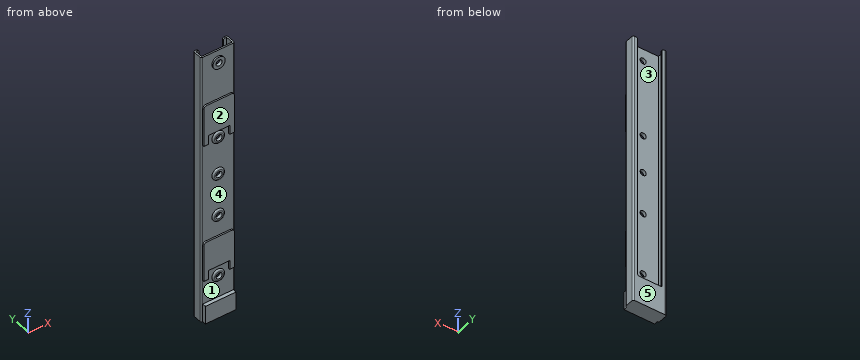
```python
from build123d import *

# Parameters (mm, degrees)
SKETCH1_W           = 11
SKETCH1_H           = 90
BOSS_EXTRUDE1_DEPTH = 3.5
CUT_EXTRUDE1_DEPTH  = 81
CUT_EXTRUDE2_DEPTH  = 6
FILLET1_R           = 0.5
FILLET2_R           = 0.5
SKETCH4_R           = 2
SKETCH4_R_2         = 1
BOSS_EXTRUDE2_DEPTH = 0.5
CUT_EXTRUDE3_START  = -1
SKETCH4_2_R         = 1
CUT_EXTRUDE3_DEPTH  = 1
FILLET3_R           = 0.5
FILLET4_R           = 1
SKETCH5_W           = 10
SKETCH5_H           = 6
BOSS_EXTRUDE3_DEPTH = 1.2


with BuildPart() as part:
    # Sketch1 → Boss-Extrude1 (new body)
    with BuildSketch(Plane(origin=(0, 0, 0), x_dir=(1, 0, 0), z_dir=(0, 1, 0))):
        Rectangle(SKETCH1_W, SKETCH1_H)
    extrude(amount=BOSS_EXTRUDE1_DEPTH)

    # Sketch2 → Cut-Extrude1 (cut)
    with BuildSketch(Plane.XY.offset(45)):
        Polygon((-4, 3.5), (-4, 3), (-5, 3), (-5, 0.5), (5, 0.5), (5, 3), (4, 3), (4, 3.5), align=None)
    extrude(amount=-CUT_EXTRUDE1_DEPTH, mode=Mode.SUBTRACT)

    # Sketch3 → Cut-Extrude2 (cut)
    with BuildSketch(Plane.XY.offset(-36)):
        Polygon((-4, 3), (4, 3), (5, 3), (5, 0.5), (-5, 0.5), (-5, 3), align=None)
    extrude(amount=-CUT_EXTRUDE2_DEPTH, mode=Mode.SUBTRACT)

    # Fillet1
    fillet1_edges = [part.edges().sort_by_distance(p)[0] for p in [
        (-5.5, 3.5, 0),
        (5.5, 3.5, 0),
        (-5.5, 0, 0),
        (5.5, 0, 0),
    ]]
    fillet(fillet1_edges, radius=FILLET1_R)

    # Fillet2
    fillet2_edges = [part.edges().sort_by_distance(p)[0] for p in [
        (4, 3.25, -36),
        (-4, 3.25, -36),
        (-4, 3.25, 45),
        (4, 3.25, 45),
    ]]
    fillet(fillet2_edges, radius=FILLET2_R)

    # Sketch4 → Boss-Extrude2 (add)
    # profile 1 of 7: a face of its own
    with BuildSketch(Plane.XZ):
        with Locations(Location((0, -31.5, 0), (0, 0, 270))):
            Circle(SKETCH4_R)
        with Locations(Location((0, -31.5, 0), (0, 0, 270))):
            Circle(SKETCH4_R_2, mode=Mode.SUBTRACT)
    # profile 2 of 7: a face of its own
    with BuildSketch(Plane.XZ):
        with Locations(Location((0, -11, 0), (0, 0, 270))):
            Circle(SKETCH4_R)
        with Locations(Location((0, -11, 0), (0, 0, 270))):
            Circle(SKETCH4_R_2, mode=Mode.SUBTRACT)
    # profile 3 of 7: a face of its own
    with BuildSketch(Plane.XZ):
        with Locations(Location((0, 3, 0), (0, 0, 270))):
            Circle(SKETCH4_R)
        with Locations(Location((0, 3, 0), (0, 0, 270))):
            Circle(SKETCH4_R_2, mode=Mode.SUBTRACT)
    # profile 4 of 7: a face of its own
    with BuildSketch(Plane.XZ):
        with Locations(Location((0, 41, 0), (0, 0, 270))):
            Circle(SKETCH4_R)
        with Locations(Location((0, 41, 0), (0, 0, 270))):
            Circle(SKETCH4_R_2, mode=Mode.SUBTRACT)
    # profile 5 of 7: a face of its own
    with BuildSketch(Plane.XZ):
        with Locations(Location((0, 15.5, 0), (0, 0, 270))):
            Circle(SKETCH4_R)
        with Locations(Location((0, 15.5, 0), (0, 0, 270))):
            Circle(SKETCH4_R_2, mode=Mode.SUBTRACT)
    # profile 6 of 7: a face of its own
    with BuildSketch(Plane.XZ):
        Polygon((5, 28.5), (-5, 28.5), (-5, 15), (-3.5, 15), (-3.5, 18), (3.5, 18), (3.5, 15), (5, 15), align=None)
    # profile 7 of 7: a face of its own
    with BuildSketch(Plane.XZ):
        Polygon((5, -18), (-5, -18), (-5, -31), (-3.5, -31), (-3.5, -28), (3.5, -28), (3.5, -31), (5, -31), align=None)
    extrude(amount=BOSS_EXTRUDE2_DEPTH)

    # Sketch4<2> → Cut-Extrude3 (cut)
    with BuildSketch(Plane.XZ.offset(CUT_EXTRUDE3_START)):
        with Locations(Location((0, -31.5, 0), (0, 0, 270))):
            Circle(SKETCH4_2_R)
        with Locations(Location((0, -11, 0), (0, 0, 270))):
            Circle(SKETCH4_2_R)
        with Locations(Location((0, 3, 0), (0, 0, 270))):
            Circle(SKETCH4_2_R)
        with Locations(Location((0, 15.5, 0), (0, 0, 270))):
            Circle(SKETCH4_2_R)
        with Locations(Location((0, 41, 0), (0, 0, 270))):
            Circle(SKETCH4_2_R)
    extrude(amount=CUT_EXTRUDE3_DEPTH, mode=Mode.SUBTRACT)

    # Fillet3
    fillet3_edges = [part.edges().sort_by_distance(p)[0] for p in [
        (0, -0.5, -29.5),
        (0, -0.5, -9),
        (0, -0.5, 5),
        (0, -0.5, 17.5),
    ]]
    fillet(fillet3_edges, radius=FILLET3_R - 0.0001)  # a hair under: the kernel refuses the full size

    # Fillet4
    fillet4_edges = [part.edges().sort_by_distance(p)[0] for p in [
        (5, -0.25, 28.5),
        (-5, -0.25, 28.5),
        (5, -0.25, -18),
        (-5, -0.25, -18),
    ]]
    fillet(fillet4_edges, radius=FILLET4_R)

    # Sketch5 → Boss-Extrude3 (add)
    with BuildSketch(Plane.XZ):
        with Locations((0, -42)):
            Rectangle(SKETCH5_W, SKETCH5_H)
    extrude(amount=BOSS_EXTRUDE3_DEPTH)


solid = part.part
```
Verification items for the finished model (mm, model axes). Face numbers are marked on the shaded views. A direction names the side the tool comes from. Coordinates: 2 decimals unless noted, no trailing zeros. Order: outer loops, then holes, each group sorted by start corner. A loop starts at its lowest first (then second) coordinate and runs counter-clockwise, first axis right, second up. Notation, with made-up numbers: (-32, -15) -> (-21, -15) arc R32 cw to (-21, 16) -> close; hole circle Ø6 at (15.25, 40.25). An arc over 180 degrees is marked (long way). Answer as CSV lines item,"result". Start each with the question number.
1) Set-up check for the marked faces 1 and 2: record each of +Z, -Z, +X, -X, +Y, -Y from which the full face is reachable in a straight line by a thin tool's end or side.
2) Cross-section at B-B, the plane y = 1.25. Record the boundary of the cut face in (x, z).
3) Release check for a two-part mould opening along Y. For the marked faces 3, 4 and 5 record: released by +Y, released by -Y, zero draft, split by the parting line, or undercut.
4) Cross-section at D-D, the plane x = 0. Give the number of separate pieces and of enclosed holes in the cut face, then the cut area to 3 significant figures.
5) Material ranges on L1, parallel to Z at x = 0, y = 0.05; L2, parallel to X at y = 1.25, z = -39; L3, parallel to X at y = -0.1, z = 3, recorded low to high. Write a range as [from, to].
6) Cross-section at A-A, the plane z = 41. Record the boundary of the cut face in (x, y).
7) Gauge pin test, flat ends, axial feed: pin 1 Ø4.5 at (x, z) = (0.5, 41.5) entering from -Y; pin 2 Ø1.3 at (y, z) = (-0.5, -41) entering from -X; pin 3 Ø3 at (x, z) = (0, -11) entering from +Y. Record the tip position at first contact, or that the pin passes through.
Conclusion:
1,face 1,"-Y"
1,face 2,"+Z, +X, -X, -Y"
2,outline,"(-5.5, -45) -> (5.5, -45) -> (5.5, 45) -> (5, 45) -> (5, -42) -> (-5, -42) -> (-5, 45) -> (-5.5, 45) -> close"
3,face 3,"undercut"
3,face 4,"released by -Y"
3,face 5,"released by +Y"
4,separate pieces,"6"
4,enclosed holes,"0"
4,area,"74.0 mm²"
5,L1,"z = [-45, -32.5], [-30.5, -12], [-10, 2], [4, 14.5], [16.5, 40], [42, 45]"
5,L2,"x = [-5.5, -5], [5, 5.5]"
5,L3,"x = [-1.99, -1], [1, 1.99]"
6,outline,"(-5.5, 0.5) arc R0.5 ccw to (-5, 0) -> (-2, 0) -> (-2, -0.5) -> (-1, -0.5) -> (-1, 0.5) -> (-5, 0.5) -> (-5, 3) -> (-4, 3) -> (-4, 3.5) -> (-5, 3.5) arc R0.5 ccw to (-5.5, 3) -> close; (1, -0.5) -> (2, -0.5) -> (2, 0) -> (5, 0) arc R0.5 ccw to (5.5, 0.5) -> (5.5, 3) arc R0.5 ccw to (5, 3.5) -> (4, 3.5) -> (4, 3) -> (5, 3) -> (5, 0.5) -> (1, 0.5) -> close"
7,pin 1,"stops at y = -0.5"
7,pin 2,"stops at x = -5.36"
7,pin 3,"stops at y = 0.5"
